Source: CAD feature listing. Evaluate the final solid. Frame: model axes, mm. A direction names the side the tool comes from. Round coordinates to 2 decimals unless told otherwise and drop trailing zeros. Write each loop counter-clockwise with the first axis right and the second up, starting at its lowest first coordinate (ties: lowest second). Pieces come first, ordered by that corner, then holes. Notation, with made-up numbers: (41.25, 21) -> (60.25, 21) arc R10 ccw to (60.25, 37) -> close; hole circle Ø9 at (0.25, -35). An arc over 180 degrees is marked (long way). Put each result on its own line as item: value.
Autodesk Inventor part; units mm, degrees
ref_plane "YZ Plane" through (0, 0, 0) normal (1, 0, 0) x (0, 1, 0)
ref_plane "XZ Plane" through (0, 0, 0) normal (0, 1, 0) x (-1, 0, 0)
ref_plane "XY Plane" through (0, 0, 0) normal (0, 0, 1) x (1, 0, 0)
sketch "Sketch1" plane through (0, 0, 0) normal (0, 0, 1) x (1, 0, 0)
  circle A0 centre (20.4823, 12.853) radius 3.1
  circle A1 centre (20.4823, 12.853) radius 10
  circle A2 centre (27.0323, 12.853) radius 2
  circle A3 centre (25.1139, 17.4846) radius 2
  circle A4 centre (20.4823, 19.403) radius 2
  circle A5 centre (15.8508, 17.4846) radius 2
  circle A6 centre (13.9323, 12.853) radius 2
  circle A7 centre (15.8508, 8.2215) radius 2
  circle A8 centre (20.4823, 6.303) radius 2
  circle A9 centre (25.1139, 8.2215) radius 2
  line L0 (15.8508, 17.4846) -> (13.9323, 12.853)
  line L1 (14.8916, 15.1688) -> (17.6183, 14.0393)
  line L2 (20.4823, 19.403) -> (25.1139, 17.4846)
  line L3 (22.7981, 18.4438) -> (21.6686, 15.717)
  line L4 (27.0323, 12.853) -> (25.1139, 8.2215)
  line L5 (26.0731, 10.5372) -> (23.3464, 11.6667)
  line L6 (15.8508, 8.2215) -> (20.4823, 6.303)
  line L7 (18.1666, 7.2622) -> (19.296, 9.989)
  circle A10 centre (20.4823, 12.853) radius 4.25
  circle A11 centre (16.5558, 14.4794) radius 0.5
  circle A12 centre (22.1087, 16.7795) radius 0.5
  circle A13 centre (24.4088, 11.2266) radius 0.5
  circle A14 centre (18.8559, 8.9265) radius 0.5
  point P0 (0, 0)
  dimension "d0" = 8.5
  dimension "d1" = 1
  dimension "d2" = 1
  dimension "d3" = 1
  dimension "d4" = 1
extrude "Extrusion1" add sketch "Sketch1" along normal blind 8.5 contours A0 L3 A12 A10 A13 L5 | A0 L1 A11 A10 A12 L3 | L5 A13 A10 A14 L7 A0 | A0 L7 A14 A10 A11 L1 | A1
sketch "Sketch2" plane through (20.4823, 12.853, 0) normal (0, 0, -1) x (-1, 0, 0)
  circle A0 centre (0, 0) radius 10.25
  circle A1 centre (1.6264, -3.9265) radius 0.5
  circle A2 centre (1.6264, -3.9265) radius 0.5
  circle A3 centre (3.9265, 1.6264) radius 0.5
  circle A4 centre (3.9265, 1.6264) radius 0.5
  circle A5 centre (-1.6264, 3.9265) radius 0.5
  circle A6 centre (-1.6264, 3.9265) radius 0.5
  circle A7 centre (-3.9265, -1.6264) radius 0.5
  circle A8 centre (-3.9265, -1.6264) radius 0.5
  circle A9 centre (6.55, 0) radius 2
  circle A10 centre (6.55, 0) radius 2
  circle A11 centre (4.6315, -4.6315) radius 2
  circle A12 centre (4.6315, -4.6315) radius 2
  circle A13 centre (0, -6.55) radius 2
  circle A14 centre (0, -6.55) radius 2
  circle A15 centre (-4.6315, -4.6315) radius 2
  circle A16 centre (-4.6315, -4.6315) radius 2
  circle A17 centre (-6.55, 0) radius 2
  circle A18 centre (-6.55, 0) radius 2
  circle A19 centre (-4.6315, 4.6315) radius 2
  circle A20 centre (-4.6315, 4.6315) radius 2
  circle A21 centre (0, 6.55) radius 2
  circle A22 centre (0, 6.55) radius 2
  circle A23 centre (4.6315, 4.6315) radius 2
  circle A24 centre (4.6315, 4.6315) radius 2
  circle A25 centre (0, 0) radius 3.1
  point P0 (20.4823, -12.853)
  dimension "d7" = 20.5
extrude "Extrusion2" add sketch "Sketch2" along normal blind 0.5
sketch "Sketch4" plane through (20.4823, 12.853, 8.5) normal (0, 0, 1) x (1, 0, 0)
  point P0 (-20.4823, -12.853)
sketch "Sketch5" plane through (20.4823, 12.853, -0.5) normal (0, 0, -1) x (-1, 0, 0)
  circle A0 centre (3.9265, 1.6264) radius 0.5
  point P0 (20.4823, -12.853)
properties part number "RimV2"
Q1. Cut plane D-D on x = 11.5. Output: boundary loops of the cut face in (y, z), and give its area (3 significant figures).
Ans:
outline: (7.92, -0.5) -> (17.79, -0.5) -> (17.79, 0) -> (17.25, 0) -> (17.25, 8.5) -> (8.46, 8.5) -> (8.46, 0) -> (7.92, 0) -> close
area: 79.7 mm^2
Q2. Pin query (flat end, axial travel): pin 1 (5 mm diameter, centred on y = 19, z = 7.5, fed in from +X); pin 2 (2 mm diameter, centred on x = 25.5, z = 1.5, fed in from -Y); pin 3 (2 mm diameter, centred on x = 27, z = 4, fed in from -Y). Return the tip coordinate at first contact, or that it passes through.
Ans:
pin 1: stops at x = 29.79
pin 2: stops at y = 3.7
pin 3: stops at y = 4.51
Q3. Reachability of faces 4 (the flat face through (18, 15, -0.5)), 5 (the cylindrical face through (18.314, 22.615, 4.19)) from +Z, -Z, +X, -X, +Y, -Y: full face, straight path, thin tool, end or side. Return the list, or none.
Ans:
face 4: -Z, +X, -X, +Y, -Y
face 5: +Z
Q4. Material intervals for line 1 (X direction, y = 16, z = 0.75); line 2 (X direction, y = 18.25, z = 2.25); line 3 (X direction, y = 18.75, z = 8), sorted ascending. Write a range as [from, to].
Ans:
line 1: x = [10.99, 14.51], [17.19, 23.77], [26.45, 29.97]
line 2: x = [12.06, 14], [17.7, 18.85], [22.12, 23.27], [26.96, 28.9]
line 3: x = [12.41, 14.3], [17.4, 18.59], [22.37, 23.57], [26.66, 28.56]
Q5. Cut plane A-A on y = 12. Output: boundary loops of the cut face in (x, z), and give its area (3 significant figures).
Ans:
outline: (10.27, -0.5) -> (12.12, -0.5) -> (12.12, 8.5) -> (10.52, 8.5) -> (10.52, 0) -> (10.27, 0) -> close; (15.74, -0.5) -> (17.5, -0.5) -> (17.5, 8.5) -> (15.74, 8.5) -> close; (23.46, -0.5) -> (25.22, -0.5) -> (25.22, 8.5) -> (23.46, 8.5) -> close; (28.84, -0.5) -> (30.7, -0.5) -> (30.7, 0) -> (30.45, 0) -> (30.45, 8.5) -> (28.84, 8.5) -> close
area: 60.8 mm^2
Q6. Cut plane B-B on z = 2. Give the number of separate pieces and of enclosed holes in the cut face, and give its area (3 significant figures).
Ans:
separate pieces: 1
enclosed holes: 13
area: 180 mm^2
Q7. Draft query along X for faces 1 (the cylindrical face through (24.039, 15.798, -0.246)), 2 (the cylindrical face through (14.97, 4.21, -0.25)), 3 (the flat face through (23, 15, 8.5)). Return one class per face: +X half, -X half, draft (parallel to the pull), parting line (faces both ways), or undercut.
Ans:
face 1: undercut
face 2: parting line
face 3: draft
Q8. Cut plane C-C on y = 5.75. Output: boundary loops of the cut face in (x, z).
Ans:
outline: (13.09, -0.5) -> (18.56, -0.5) -> (18.56, 8.5) -> (13.44, 8.5) -> (13.44, 0) -> (13.09, 0) -> close; (22.4, -0.5) -> (27.87, -0.5) -> (27.87, 0) -> (27.52, 0) -> (27.52, 8.5) -> (22.4, 8.5) -> close
